Model file for the job. Use its own axes, mm. A direction names the side the tool comes from. Round coordinates to 2 decimals unless told otherwise and drop trailing zeros. Write each loop counter-clockwise with the first axis right and the second up, starting at its lowest first coordinate (ties: lowest second). Pieces come first, ordered by that corner, then holes. Notation, with made-up numbers: (80.5, 7) - (97.5, 7) arc R26 ccw to (97.5, 29) - close; hole circle Ø11 at (-17, -36). An arc over 180 degrees is marked (long way). One line per item, written item: value.
from build123d import *

# Parameters (mm, degrees)
SKETCH1_W           = 8.128
SKETCH1_H           = 8.128
BOSS_EXTRUDE1_DEPTH = 4.445
SKETCH2_W           = 6.35
SKETCH2_H           = 6.35
CUT_EXTRUDE1_DEPTH  = 4.064
SKETCH3_R           = 2.159
CUT_EXTRUDE2_DEPTH  = 8.265687648
BOSS_EXTRUDE2_START = 6.35
SKETCH4_R           = 3.175
SKETCH4_R_2         = 2.159
BOSS_EXTRUDE2_DEPTH = 6.35


with BuildPart() as part:
    # Sketch1 → Boss-Extrude1 (new body)
    with BuildSketch(Plane(origin=(0, 0, 0), x_dir=(1, 0, 0), z_dir=(0, 1, 0))):
        Rectangle(SKETCH1_W, SKETCH1_H)
    extrude(amount=-BOSS_EXTRUDE1_DEPTH)

    # Sketch2 → Cut-Extrude1 (cut)
    with BuildSketch(Plane.XZ.offset(4.445)):
        Rectangle(SKETCH2_W, SKETCH2_H)
    extrude(amount=-CUT_EXTRUDE1_DEPTH, mode=Mode.SUBTRACT)

    # Sketch3 → Cut-Extrude2 (cut, through all)
    with BuildSketch(Plane(origin=(0, 0, 0), x_dir=(1, 0, 0), z_dir=(0, 1, 0))):
        with Locations(Location((0, 0, 0), (0, 0, 270))):
            Circle(SKETCH3_R)
    extrude(amount=-CUT_EXTRUDE2_DEPTH, mode=Mode.SUBTRACT)

    # Sketch4 → Boss-Extrude2 (add)
    with BuildSketch(Plane(origin=(0, 0, 0), x_dir=(1, 0, 0), z_dir=(0, 1, 0)).offset(BOSS_EXTRUDE2_START)):
        with Locations(Location((0, 0, 0), (0, 0, 270))):
            Circle(SKETCH4_R)
        with Locations(Location((0, 0, 0), (0, 0, 270))):
            Circle(SKETCH4_R_2, mode=Mode.SUBTRACT)
    extrude(amount=-BOSS_EXTRUDE2_DEPTH)


solid = part.part
1. Tool access for faces 1 (the face through (-3.175, -2, 0)), 2 (the face through (-1.93, 3.22, -2.52)), 3 (the face through (3.6, -4.445, -0.1)): list every direction of +Z, -Z, +X, -X, +Y, -Y with a clear straight run to the whole face (end or side of a thin tool).
Report:
face 1: -Y
face 2: +Y
face 3: +Z, -Z, +X, -X, -Y
2. Band-saw the part on D-D on z = 2.75. Write the cut outline in (x, y) (3 decimals), plus the area to 3 significant figures.
Report:
outline: (-4.064, -4.445) - (-3.175, -4.445) - (-3.175, -0.381) - (3.175, -0.381) - (3.175, -4.445) - (4.064, -4.445) - (4.064, 0) - (1.587, 0) - (1.587, 6.35) - (-1.587, 6.35) - (-1.587, 0) - (-4.064, 0) - close
area: 30.5 mm²
3. Band-saw the part on C-C on y = -0.25. Write the cut outline in (x, z), plus the area to 3 significant figures.
Report:
outline: (-4.06, -4.06) - (4.06, -4.06) - (4.06, 4.06) - (-4.06, 4.06) - close; hole circle Ø4.32 at (0, 0)
area: 51.4 mm²
4. Band-saw the part on B-B on z = 0. Write the cut outline in (x, y) (3 decimals), plus the area to 3 significant figures.
Report:
outline: (-4.064, -4.445) - (-3.175, -4.445) - (-3.175, -0.381) - (-2.159, -0.381) - (-2.159, 6.35) - (-3.175, 6.35) - (-3.175, 0) - (-4.064, 0) - close; (2.159, -0.381) - (3.175, -0.381) - (3.175, -4.445) - (4.064, -4.445) - (4.064, 0) - (3.175, 0) - (3.175, 6.35) - (2.159, 6.35) - close
area: 21.6 mm²
5. Band-saw the part on A-A on x = 0. Write the cut outline in (y, z) (3 decimals).
Report:
outline: (-4.445, -4.064) - (0, -4.064) - (0, -3.175) - (6.35, -3.175) - (6.35, -2.159) - (-0.381, -2.159) - (-0.381, -3.175) - (-4.445, -3.175) - close; (-4.445, 3.175) - (-0.381, 3.175) - (-0.381, 2.159) - (6.35, 2.159) - (6.35, 3.175) - (0, 3.175) - (0, 4.064) - (-4.445, 4.064) - close
6. Mould opens along X. For faces 4 (the face through (-3, 0, -2)), 5 (the face through (-0.8, -0.381, 2.2)), 6 (the face through (4.064, -2, 0)) say: released by +X, released by -X, zero draft, split by the parting line, or undercut.
Report:
face 4: zero draft
face 5: undercut
face 6: released by +X
7. Wall check: probe 1 along X at (y, z) = (4, 0) (3 decimals); probe 2 along X at (y, z) = (-2.75, 0.5) (3 decimals). Give the ranges that are in metal, low to high. Write a range as [from, to].
Report:
probe 1: [-3.175, -2.159], [2.159, 3.175]
probe 2: [-4.064, -3.175], [3.175, 4.064]
8. Drop flat-ended pins along their axis: pin 1 (1 mm diameter, centred on x = 0.5, y = 3.5, fed in from -Z) (3 decimals); pin 2 (1.5 mm diameter, centred on x = 3, y = 3.5, fed in from +Z). Give the stop position or say it passes through.
Report:
pin 1: z = -3.175
pin 2: z = 2.24
